Autodesk Inventor part; units mm, degrees
ref_plane "YZ Plane" through (0, 0, 0) normal (1, 0, 0) x (0, 1, 0)
ref_plane "XZ Plane" through (0, 0, 0) normal (0, 1, 0) x (-1, 0, 0)
ref_plane "XY Plane" through (0, 0, 0) normal (0, 0, 1) x (1, 0, 0)
sketch "Sketch1" plane through (0, 0, 0) normal (0, 0, 1) x (1, 0, 0)
  circle A0 centre (0, 0) radius 1.8
  circle A1 centre (0, 0) radius 17
  circle A2 centre (0, 0) radius 8.5
  circle A3 centre (0, 0) radius 24
  circle A4 centre (20.75, 0) radius 1.8
  circle A5 centre (14.6725, 14.6725) radius 1.8
  circle A6 centre (0, 20.75) radius 1.8
  circle A7 centre (-14.6725, 14.6725) radius 1.8
  circle A8 centre (-20.75, 0) radius 1.8
  circle A9 centre (-14.6725, -14.6725) radius 1.8
  circle A10 centre (0, -20.75) radius 1.8
  circle A11 centre (14.6725, -14.6725) radius 1.8
  dimension "d0" = 3.6
  dimension "d1" = 34
  dimension "d2" = 17
  dimension "d3" = 48
  dimension "d4" = 3.6
  dimension "d5" = 20.75
  dimension "d8" = 360
extrude "Extrusion1" add sketch "Sketch1" along normal blind 2 contours A1 | A2 | A3
extrude "Extrusion2" add sketch "Sketch1" along normal blind 10 contours A3
fillet "Fillet1" radius 2 1 edges at (-17, 0, 2)
properties part number "MoldeA"
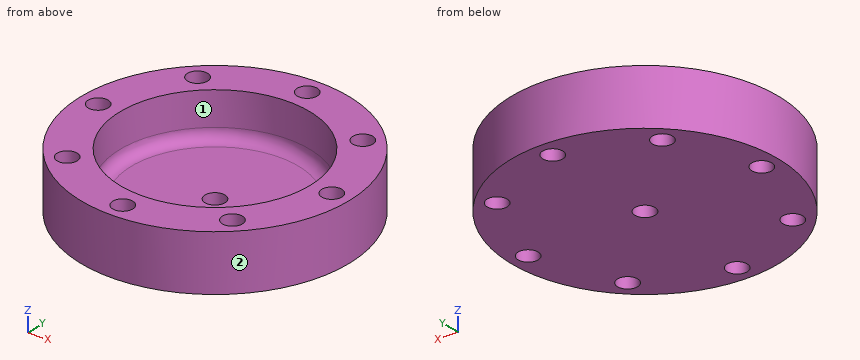
Verification items for the finished model (mm, model axes). Face numbers are marked on the shaded views. A direction names the side the tool comes from. Give positions to 0.01 mm unless a question says otherwise; leave off trailing zeros. Order: outer loops, then holes, each group sorted by start corner. A loop starts at its lowest first (then second) coordinate and runs counter-clockwise, first axis right, second up. Notation, with made-up numbers: M -36.75,-28.5 L -28.75,-28.5 A8 cw -28.75,-23.5 Z; hole C 15.25,80.25 d8. An arc over 180 degrees is marked long. Answer in a Markdown table with one row per item. Add a question column.
Item 1: Section check A-A, the plane y = 0. Enter the section's corners in (x, z), and give its area (3 significant figures).
Item 2: Section check C-C, the plane x = -20.75. Enter the section's corners in (y, z), and give its area (3 significant figures).
Item 3: Gauge pin test, flat ends, axial feed: pin 1 (1 mm diameter, centred on y = -11.5, z = 4, fed in from +X); pin 2 (1.5 mm diameter, centred on x = -1.5, z = 6, fed in from -Y); pin 3 (6 mm diameter, centred on x = -20.75, y = 0, fed in from +Z); pin 4 (5 mm diameter, centred on x = 19, z = 6, fed in from +Y). Record the tip position at first contact, or that the pin passes through.
Item 4: Tool access check on the marked faces 1 and 2. Record the directions out of +Z, -Z, +X, -X, +Y, -Y that give a thin tool (end or side, any length) a straight path to the whole face; none if there is none.
Item 5: Scan lines: probe 1 along Y at (x, z) = (0, 8.25); probe 2 along Y at (x, z) = (14, 4.5); probe 3 along Y at (x, z) = (-6.5, 3.5). Record each from-to range of solid material in increasing order. Write a range as from..to.
Filled sheet:
| question | item | result |
|---|---|---|
| 1 | outline | M -24,0 L -22.55,0 L -22.55,10 L -24,10 Z; M -18.95,0 L -1.8,0 L -1.8,2 L -15,2 A2 cw -17,4 L -17,10 L -18.95,10 Z; M 1.8,0 L 18.95,0 L 18.95,10 L 17,10 L 17,4 A2 cw 15,2 L 1.8,2 Z; M 22.55,0 L 24,0 L 24,10 L 22.55,10 Z |
| 1 | area | 131 mm^2 |
| 2 | outline | M -12.06,0 L -1.8,0 L -1.8,10 L -12.06,10 Z; M 1.8,0 L 12.06,0 L 12.06,10 L 1.8,10 Z |
| 2 | area | 205 mm^2 |
| 3 | pin 1 | stops at x = 21.33 |
| 3 | pin 2 | stops at y = -23.99 |
| 3 | pin 3 | stops at z = 10 |
| 3 | pin 4 | stops at y = 17.43 |
| 4 | face 1 | +Z |
| 4 | face 2 | +Z, -Z |
| 5 | probe 1 | y = -24..-22.55, -18.95..-17, 17..18.95, 22.55..24 |
| 5 | probe 2 | y = -19.49..-16.34, -13..-9.64, 9.64..13, 16.34..19.49 |
| 5 | probe 3 | y = -23.1..-15.64, 15.64..23.1 |
